```python
from build123d import *

# Parameters (mm, degrees)
SKETCH1_R               = 1.500000001
SKETCH1_R_2             = 1.5
BOSS_EXTRUDE2_DEPTH     = 4
SKETCH1_4_W             = 32
SKETCH1_4_H             = 35
SKETCH1_4_R             = 6.100000001
BOSS_EXTRUDE3_DEPTH     = 20
SKETCH2_R               = 1.5
CUT_EXTRUDE3_DEPTH      = 1
CUT_EXTRUDE3_DEPTH_BACK = 33
CUT_EXTRUDE4_DEPTH      = 5
CUT_EXTRUDE5_START      = -32
CUT_EXTRUDE5_DEPTH      = 5
CUT_EXTRUDE6_DEPTH      = 25
BOSS_EXTRUDE5_DEPTH     = 12.5
SKETCH7_R               = 1.4
CUT_EXTRUDE7_DEPTH      = 20
BOSS_EXTRUDE6_START     = -32
BOSS_EXTRUDE6_DEPTH     = 10
CUT_EXTRUDE8_DEPTH      = 43
SKETCH9_R               = 1.4
SKETCH9_W               = 32
SKETCH9_H               = 28
SKETCH9_R_2             = 1.500000001
BOSS_EXTRUDE7_DEPTH     = 2
SKETCH1_8_W             = 32
SKETCH1_8_H             = 27.5
SKETCH1_8_R             = 1.500000001
SKETCH1_8_R_2           = 1.5
CUT_EXTRUDE9_DEPTH      = 4
SKETCH11_W              = 1
SKETCH11_H              = 28
CUT_EXTRUDE13_DEPTH     = 27
CUT_EXTRUDE10_DEPTH     = 55.5


with BuildPart() as part:
    # Sketch1 → Boss-Extrude2 (new body)
    with BuildSketch(Plane.XY):
        Polygon((-16, 49), (-16, -46.5), (-14.969293645, -46.5), (-14.969293645, -42.160880121), (-15.92820323, -40.5), (-12.464101615, -34.5), (-5.535898385, -34.5), (-2.07179677, -40.5), (-5.535898385, -46.5), (5.535898385, -46.5), (2.090853862, -40.533007852), (5.457729166, -34.432863746), (12.425340481, -34.432863746), (15.909146138, -40.466992148), (15, -42.114193768), (15, -46.5), (16, -46.5), (16, 49), align=None)
        with Locations((10, 10)):
            Circle(SKETCH1_R, mode=Mode.SUBTRACT)
        with Locations((-10, -10)):
            Circle(SKETCH1_R, mode=Mode.SUBTRACT)
        with Locations((10, -10)):
            Circle(SKETCH1_R, mode=Mode.SUBTRACT)
        with Locations((-10, 10)):
            Circle(SKETCH1_R, mode=Mode.SUBTRACT)
        with Locations((0, -43.5)):
            Circle(SKETCH1_R_2, mode=Mode.SUBTRACT)
        with Locations((-8.5, -31.5)):
            Circle(SKETCH1_R_2, mode=Mode.SUBTRACT)
        with Locations((8.5, -31.5)):
            Circle(SKETCH1_R_2, mode=Mode.SUBTRACT)
    extrude(amount=BOSS_EXTRUDE2_DEPTH)

    # Sketch1<4> → Boss-Extrude3 (add)
    with BuildSketch(Plane.XY):
        with Locations((0, 31.5)):
            Rectangle(SKETCH1_4_W, SKETCH1_4_H)
        Polygon((0, 36.969655115), (9.5, 31.484827557), (9.5, 20.515172443), (0, 15.030344885), (-9.5, 20.515172443), (-9.5, 31.484827557), align=None, mode=Mode.SUBTRACT)
        Polygon((9.5, 31.484827557), (9.5, 20.515172443), (0, 15.030344885), (-9.5, 20.515172443), (-9.5, 31.484827557), (0, 36.969655115), align=None)
        with Locations((0, 26)):
            Circle(SKETCH1_4_R, mode=Mode.SUBTRACT)
        with Locations((0, 26)):
            Circle(SKETCH1_4_R)
    extrude(amount=-BOSS_EXTRUDE3_DEPTH)

    # Sketch2 → Cut-Extrude3 (cut, two sides)
    with BuildSketch(Plane.ZY.offset(16)) as cut_extrude3_sk:
        with Locations((-1.580023732, 25.999827557)):
            Circle(SKETCH2_R)
    extrude(amount=CUT_EXTRUDE3_DEPTH, mode=Mode.SUBTRACT)
    extrude(cut_extrude3_sk.sketch, amount=-CUT_EXTRUDE3_DEPTH_BACK, mode=Mode.SUBTRACT)

    # Sketch3 → Cut-Extrude4 (cut)
    with BuildSketch(Plane.ZY.offset(16)):
        with BuildLine():
            Line((0.716979622, 28.369168308), (-1.239134605, 30.265561192))
            ThreePointArc((-1.239134605, 30.265561192), (-1.539975782, 30.904899692), (-1.343104133, 31.583501701))
            ThreePointArc((-1.343104133, 31.583501701), (2.506062966, 39.867185425), (2.670991263, 49))
            Line((2.670991263, 49), (-20, 49))
            Line((-20, 49), (-20, 22.778106647))
            ThreePointArc((-20, 22.778106647), (-13.472070231, 23.458477945), (-7.432949471, 26.028651597))
            ThreePointArc((-7.432949471, 26.028651597), (-6.799957072, 26.171029415), (-6.212814046, 25.894960789))
            Line((-6.212814046, 25.894960789), (-3.877027086, 23.630486807))
            Line((-3.877027086, 23.630486807), (0.716979622, 28.369168308))
        make_face()
        with BuildLine():
            ThreePointArc((-3.877027086, 23.630486807), (0.789317018, 23.702824203), (0.716979622, 28.369168308))
            Line((0.716979622, 28.369168308), (-3.877027086, 23.630486807))
        make_face()
    extrude(amount=-CUT_EXTRUDE4_DEPTH, mode=Mode.SUBTRACT)

    # Sketch3<4> → Cut-Extrude5 (cut)
    with BuildSketch(Plane.ZY.offset(16).offset(CUT_EXTRUDE5_START)):
        with BuildLine():
            Line((0.716979622, 28.369168308), (-1.239134605, 30.265561192))
            ThreePointArc((-1.239134605, 30.265561192), (-1.539975782, 30.904899692), (-1.343104133, 31.583501701))
            ThreePointArc((-1.343104133, 31.583501701), (2.506062966, 39.867185425), (2.670991263, 49))
            Line((2.670991263, 49), (-20, 49))
            Line((-20, 49), (-20, 22.778106647))
            ThreePointArc((-20, 22.778106647), (-13.472070231, 23.458477945), (-7.432949471, 26.028651597))
            ThreePointArc((-7.432949471, 26.028651597), (-6.799957072, 26.171029415), (-6.212814046, 25.894960789))
            Line((-6.212814046, 25.894960789), (-3.877027086, 23.630486807))
            Line((-3.877027086, 23.630486807), (0.716979622, 28.369168308))
        make_face()
        with BuildLine():
            ThreePointArc((-3.877027086, 23.630486807), (0.789317018, 23.702824203), (0.716979622, 28.369168308))
            Line((0.716979622, 28.369168308), (-3.877027086, 23.630486807))
        make_face()
    extrude(amount=CUT_EXTRUDE5_DEPTH, mode=Mode.SUBTRACT)

    # Sketch5 → Cut-Extrude6 (cut, through all)
    with BuildSketch(Plane.XY.offset(4)):
        Polygon((-14.969293645, -42.160880121), (-15.92820323, -40.5), (-16, -40.500074436), (-16, -46.5), (-14.969293645, -46.5), align=None)
        Polygon((15, -42.114193768), (15.909146138, -40.466992148), (10.36687247, -40.472738184), (10.36687247, -46.5), (15, -46.5), align=None)
        Polygon((16, -40.466897954), (15.909146138, -40.466992148), (15, -42.114193768), (15, -46.5), (16, -46.5), align=None)
        Polygon((17.825288522, -40.465005559), (16, -40.466897954), (16, -46.5), (17.916172301, -46.5), align=None)
    extrude(amount=-CUT_EXTRUDE6_DEPTH, mode=Mode.SUBTRACT)

    # Sketch8 → Boss-Extrude5 (add)
    with BuildSketch(Plane.ZY.offset(16)):
        with BuildLine():
            ThreePointArc((-1.343104133, 31.583501701), (-1.539975782, 30.904899692), (-1.239134605, 30.265561192))
            Line((-1.239134605, 30.265561192), (0.716979622, 28.369168308))
            ThreePointArc((0.716979622, 28.369168308), (0.789317018, 23.702824203), (-3.877027086, 23.630486807))
            Line((-3.877027086, 23.630486807), (-6.212814046, 25.894960789))
            ThreePointArc((-6.212814046, 25.894960789), (-6.799957072, 26.171029415), (-7.432949471, 26.028651597))
            ThreePointArc((-7.432949471, 26.028651597), (-13.472070231, 23.458477945), (-20, 22.778106647))
            Line((-20, 22.778106647), (-20, 14))
            Line((-20, 14), (0, 14))
            Line((0, 14), (4, 14))
            Line((4, 14), (4, 49))
            Line((4, 49), (2.670991263, 49))
            ThreePointArc((2.670991263, 49), (2.506062966, 39.867185425), (-1.343104133, 31.583501701))
        make_face()
    extrude(amount=BOSS_EXTRUDE5_DEPTH)

    # Sketch7 → Cut-Extrude7 (cut)
    with BuildSketch(Plane.XY.offset(4)):
        with Locations((-13.5, 37.75)):
            Circle(SKETCH7_R)
        with Locations((-23.5, 37.75)):
            Circle(SKETCH7_R)
    extrude(amount=-CUT_EXTRUDE7_DEPTH, mode=Mode.SUBTRACT)

    # Sketch8<3> → Boss-Extrude6 (add)
    with BuildSketch(Plane.ZY.offset(16).offset(BOSS_EXTRUDE6_START)):
        with BuildLine():
            ThreePointArc((-1.343104133, 31.583501701), (-1.539975782, 30.904899692), (-1.239134605, 30.265561192))
            Line((-1.239134605, 30.265561192), (0.716979622, 28.369168308))
            ThreePointArc((0.716979622, 28.369168308), (0.789317018, 23.702824203), (-3.877027086, 23.630486807))
            Line((-3.877027086, 23.630486807), (-6.212814046, 25.894960789))
            ThreePointArc((-6.212814046, 25.894960789), (-6.799957072, 26.171029415), (-7.432949471, 26.028651597))
            ThreePointArc((-7.432949471, 26.028651597), (-13.472070231, 23.458477945), (-20, 22.778106647))
            Line((-20, 22.778106647), (-20, 14))
            Line((-20, 14), (0, 14))
            Line((0, 14), (4, 14))
            Line((4, 14), (4, 49))
            Line((4, 49), (2.670991263, 49))
            ThreePointArc((2.670991263, 49), (2.506062966, 39.867185425), (-1.343104133, 31.583501701))
        make_face()
    extrude(amount=-BOSS_EXTRUDE6_DEPTH)

    # Sketch8<4> → Cut-Extrude8 (cut, through all)
    with BuildSketch(Plane.ZY.offset(16)):
        with BuildLine():
            ThreePointArc((-1.343104133, 31.583501701), (-4.126373378, 28.519223025), (-7.432949471, 26.028651597))
            ThreePointArc((-7.432949471, 26.028651597), (-13.472070231, 23.458477945), (-20, 22.778106647))
            Line((-20, 22.778106647), (-20, 49))
            Line((-20, 49), (2.670991263, 49))
            ThreePointArc((2.670991263, 49), (2.506062966, 39.867185425), (-1.343104133, 31.583501701))
        make_face()
    extrude(amount=-CUT_EXTRUDE8_DEPTH, mode=Mode.SUBTRACT)

    # Sketch9 → Boss-Extrude7 (add)
    with BuildSketch(Plane.XY.offset(4)):
        Polygon((26, 14), (26, 49), (-28.5, 49), (-28.5, 14), (-16, 14), (16, 14), align=None)
        with Locations((-23.5, 37.75)):
            Circle(SKETCH9_R, mode=Mode.SUBTRACT)
        with Locations((-13.5, 37.75)):
            Circle(SKETCH9_R, mode=Mode.SUBTRACT)
        Rectangle(SKETCH9_W, SKETCH9_H)
        with Locations((-10, -10)):
            Circle(SKETCH9_R_2, mode=Mode.SUBTRACT)
        with Locations((-10, 10)):
            Circle(SKETCH9_R_2, mode=Mode.SUBTRACT)
        with Locations((10, -10)):
            Circle(SKETCH9_R_2, mode=Mode.SUBTRACT)
        with Locations((10, 10)):
            Circle(SKETCH9_R_2, mode=Mode.SUBTRACT)
    extrude(amount=BOSS_EXTRUDE7_DEPTH)

    # Sketch1<8> → Cut-Extrude9 (cut)
    with BuildSketch(Plane.XY):
        with Locations((0, 0.25)):
            Rectangle(SKETCH1_8_W, SKETCH1_8_H)
        with Locations((-10, 10)):
            Circle(SKETCH1_8_R, mode=Mode.SUBTRACT)
        with Locations((10, 10)):
            Circle(SKETCH1_8_R, mode=Mode.SUBTRACT)
        with Locations((10, -10)):
            Circle(SKETCH1_8_R, mode=Mode.SUBTRACT)
        with Locations((-10, -10)):
            Circle(SKETCH1_8_R, mode=Mode.SUBTRACT)
        Polygon((15, -13.5), (-14.969293645, -13.5), (-14.969293645, -38.839119879), (-12.464101615, -34.5), (-5.535898385, -34.5), (-2.07179677, -40.5), (-5.535898385, -46.5), (5.535898385, -46.5), (2.090853862, -40.533007852), (5.457729166, -34.432863746), (12.425340481, -34.432863746), (15, -38.892304845), align=None)
        with Locations((-8.5, -31.5)):
            Circle(SKETCH1_8_R_2, mode=Mode.SUBTRACT)
        with Locations((0, -43.5)):
            Circle(SKETCH1_8_R_2, mode=Mode.SUBTRACT)
        with Locations((8.5, -31.5)):
            Circle(SKETCH1_8_R_2, mode=Mode.SUBTRACT)
        Polygon((-14.969293645, -13.5), (-16, -13.5), (-16, -46.5), (-14.969293645, -46.5), (-14.969293645, -42.160880121), (-15.92820323, -40.5), (-14.969293645, -38.839119879), align=None)
        Polygon((16, -46.5), (16, -13.5), (15, -13.5), (15, -38.892304845), (15.909146138, -40.466992148), (15, -42.114193768), (15, -46.5), align=None)
    extrude(amount=CUT_EXTRUDE9_DEPTH, mode=Mode.SUBTRACT)

    # Sketch11 → Cut-Extrude13 (cut, through all)
    with BuildSketch(Plane.XY.offset(6)):
        with Locations((-15.5, 0)):
            Rectangle(SKETCH11_W, SKETCH11_H)
        with Locations((15.5, 0)):
            Rectangle(SKETCH11_W, SKETCH11_H)
    extrude(amount=-CUT_EXTRUDE13_DEPTH, mode=Mode.SUBTRACT)

    # Sketch10 → Cut-Extrude10 (cut, through all)
    with BuildSketch(Plane.ZY.offset(28.5)):
        with BuildLine():
            ThreePointArc((-12, 23.89439883), (-15.948490895, 22.967108487), (-20, 22.778106647))
            Line((-20, 22.778106647), (-20, 14))
            Line((-20, 14), (-12, 14))
            Line((-12, 14), (-12, 23.89439883))
        make_face()
    extrude(amount=-CUT_EXTRUDE10_DEPTH, mode=Mode.SUBTRACT)


solid = part.part
```
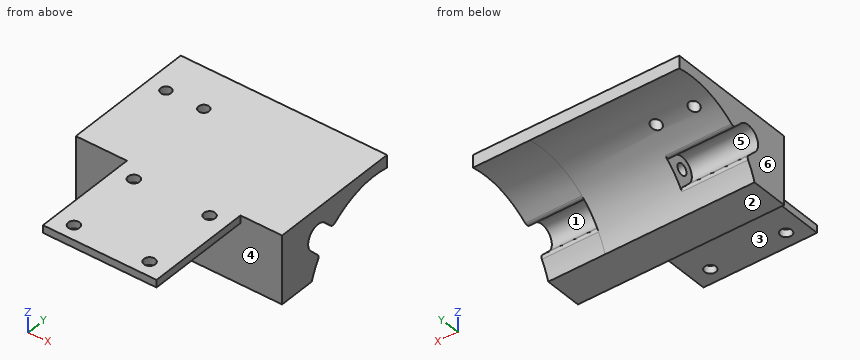
Can you work these out from the model? Positions are in its coordinate system, mm. Face numbers are marked on the shaded views. A direction names the side the tool comes from. Coordinates: 2 decimals unless noted, no trailing zeros. Write each loop counter-clockwise with the first axis right and the second up, starting at its lowest first coordinate (ties: lowest second). Pieces come first, ordered by that corner, then holes. Notation, with made-up numbers: (78.25, -37.5) - (103.25, -37.5) arc R12 ccw to (103.25, -32.5) - close; hole circle Ø3 at (-13, 59.25). An arc over 180 degrees is marked (long way). Return JSON: item names as keys, results as strings.
Q1. If we section it at B-B (x = 10): Please give me the cut outline in (y, z), then the cut area to 3 significant figures.
Computed values:
{"outline": "(-14, 4) - (-11.5, 4) - (-11.5, 6) - (-14, 6) - close; (-8.5, 4) - (8.5, 4) - (8.5, 6) - (-8.5, 6) - close; (11.5, 4) - (14, 4) - (14, -12) - (23.89, -12) arc R22.07 cw to (49, 2.67) - (49, 6) - (11.5, 6) - close; hole circle Ø3 at (26, -1.58)", "area": "374 mm2"}
Q2. If we section it at A-A (y = 10): Please give me the cut outline in (x, z).
Computed values:
{"outline": "(-15, 4) - (-11.5, 4) - (-11.5, 6) - (-15, 6) - close; (-8.5, 4) - (8.5, 4) - (8.5, 6) - (-8.5, 6) - close; (11.5, 4) - (15, 4) - (15, 6) - (11.5, 6) - close"}
Q3. I'm going to push flat-ended pins straight in: pin 1 Ø2.5 at (x, y) = (10, -10) entering from +Z; pin 2 Ø1 at (y, z) = (1, 5) entering from +X; pin 3 Ø2.5 at (y, z) = (28, -4.5) entering from +X; pin 4 Ø4 at (x, y) = (-10, 10) entering from -Z. Where does each tip first touch, or does it pass through?
Computed values:
{"pin 1": "passes through", "pin 2": "stops at x = 15", "pin 3": "stops at x = 11", "pin 4": "stops at z = 4"}
Q4. On a 3-axis mill with a long thin cutter (end or side, diameter ignored), from which of +Z, -Z, +X, -X, +Y, -Y can I reach the whole of each face in a straight line? I mean the marked faces 1, 2 and 3. Say none if no direction works.
Computed values:
{"face 1": "+X", "face 2": "-Z, +X, -X, +Y, -Y", "face 3": "-Z, +X, -X, -Y"}
Q5. Please list where these lines run through material, in increasing order: L1, parallel to X at y = 37.75, z = 3.2; L2, parallel to Y at x = 10, z = 4.6; L3, parallel to Z at x = -11, y = 45. Write a range as from..to.
Computed values:
{"L1": "x = -28.5..-24.9, -22.1..-14.9, -12.1..26", "L2": "y = -14..-11.5, -8.5..8.5, 11.5..49", "L3": "z = 3.07..6"}
Q6. If we section it at C-C (x = -23): Please give me the cut outline in (y, z).
Computed values:
{"outline": "(14, -12) - (23.89, -12) arc R22.07 cw to (26.03, -7.43) arc R1 ccw to (25.89, -6.21) - (23.63, -3.88) arc R3.3 cw to (28.37, 0.72) - (30.27, -1.24) arc R1 ccw to (31.58, -1.34) arc R22.07 cw to (36.44, 1.42) - (36.44, 6) - (14, 6) - close; (39.06, 2.3) arc R22.07 cw to (49, 2.67) - (49, 6) - (39.06, 6) - close"}
Q7. If we section it at D-D (y = 37.75): Please give me the cut outline in (x, z).
Computed values:
{"outline": "(-28.5, 1.91) - (-24.9, 1.91) - (-24.9, 6) - (-28.5, 6) - close; (-22.1, 1.91) - (-14.9, 1.91) - (-14.9, 6) - (-22.1, 6) - close; (-12.1, 1.91) - (26, 1.91) - (26, 6) - (-12.1, 6) - close"}
Q8. Thinking about a two-plate mould opening in Y: for the marked faces 4, 5 and 6, which applies, +Y half, -Y half, draft (parallel to the pull), parting line (faces both ways), or undercut?
Computed values:
{"face 4": "-Y half", "face 5": "undercut", "face 6": "draft"}
